The figure shows three views and two pictorial views of one solid part (mm, origin at its lowest corner). Answer the questions. A direction names the side the tool comes from. Round coordinates to 2 decimals unless told otherwise and drop trailing zeros. Write each loop counter-clockwise with the first axis right and the second up, starting at its lowest first coordinate (ties: lowest second). Pieces come first, ordered by that corner, then holes.
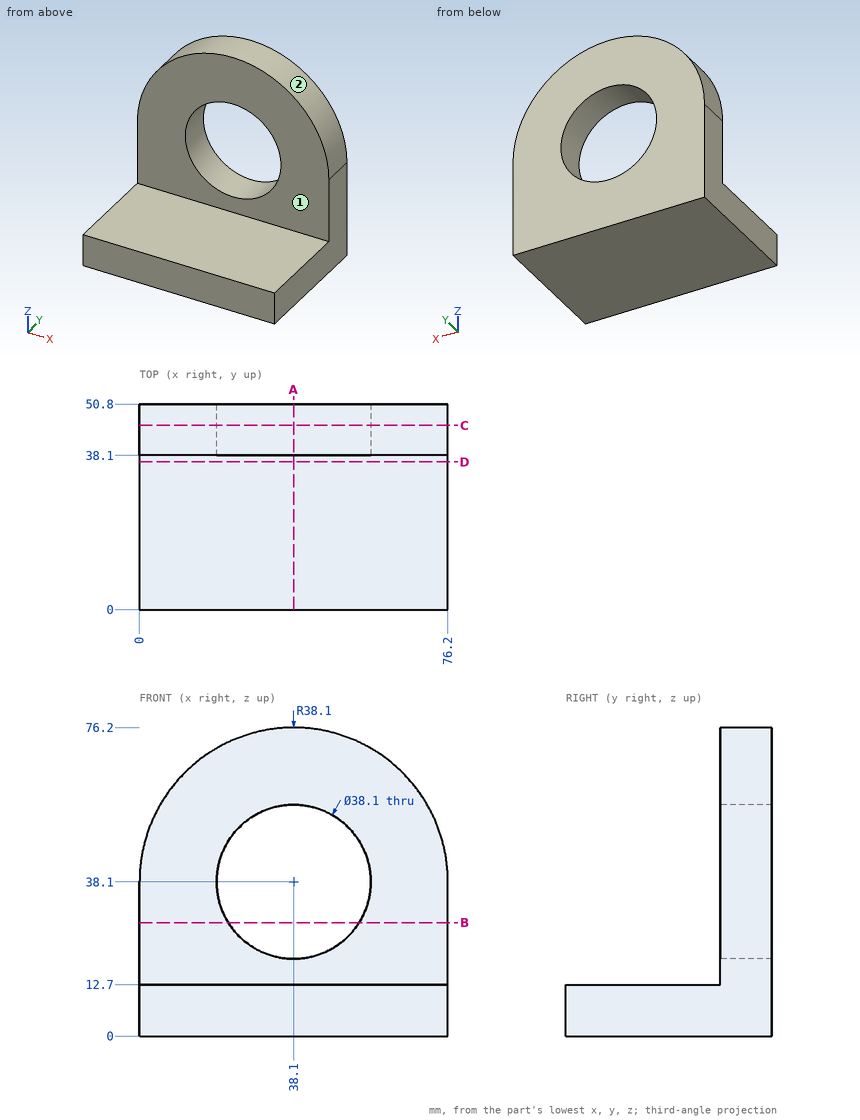
Q1. Section B-B (z = 28) is taken. Determine the outline of the cut face in (x, y), then the cut area to 3 significant figures.
Verdict:
outline: (0, 38.1) - (21.95, 38.1) - (21.95, 50.8) - (0, 50.8) - close; (54.25, 38.1) - (76.2, 38.1) - (76.2, 50.8) - (54.25, 50.8) - close
area: 557 mm2
Q2. Flat-ended cylindrical pins translate along their axes: pin 1 Ø1 at (x, z) = (66.5, 65.5) entering from -Y; pin 2 Ø8 at (x, z) = (26, 50) entering from -Y. Find the tip coordinate at first contact, or state that the pin passes through.
Verdict:
pin 1: passes through
pin 2: stops at y = 38.1
Q3. Section D-D (y = 36.5) is taken. Determine the outline of the cut face in (x, z).
Verdict:
outline: (0, 0) - (76.2, 0) - (76.2, 12.7) - (0, 12.7) - close
Q4. Section C-C (y = 45.5) is taken. Determine the outline of the cut face in (x, z), then the cut area to 3 significant figures.
Verdict:
outline: (0, 0) - (76.2, 0) - (76.2, 38.1) arc R38.1 ccw to (0, 38.1) - close; hole circle Ø38.1 at (38.1, 38.1)
area: 4,040 mm2
Q5. Section A-A (x = 38.1) is taken. Determine the outline of the cut face in (y, z), then the cut area to 3 significant figures.
Verdict:
outline: (0, 0) - (50.8, 0) - (50.8, 19.05) - (38.1, 19.05) - (38.1, 12.7) - (0, 12.7) - close; (38.1, 57.15) - (50.8, 57.15) - (50.8, 76.2) - (38.1, 76.2) - close
area: 968 mm2
Q6. Straight lines are drawn through the part: probe 1 along X at (y, z) = (42.25, 38.1); probe 2 along Z at (x, y) = (6, 26.5). For each, find the intervals that lie inside material, in ascending order.
Verdict:
probe 1: x = 0 to 19.05, 57.15 to 76.2
probe 2: z = 0 to 12.7
Q7. Which of the six approach directions +Z, -Z, +X, -X, +Y, -Y give full straight-line access (tool end or side, diameter ignored) to the marked faces 1 and 2?
Verdict:
face 1: +Z, +X, -X, -Y
face 2: +Z, +Y, -Y
